Part model, mm, in its own coordinate system. A direction names the side the tool comes from. Coordinates: 2 decimals unless noted, no trailing zeros. Write each loop counter-clockwise with the first axis right and the second up, starting at its lowest first coordinate (ties: lowest second). Pieces come first, ordered by that corner, then holes. Notation, with made-up numbers: (-39.5, 54.5) -> (-4.5, 54.5) arc R21 ccw to (-4.5, 73.5) -> close; hole circle Ø6 at (74, -34). An arc over 180 degrees is marked (long way). Write item = value, one per line. Start each with the question number.
Q1. Band-saw the part on C-C, the plane z = 45. List the corners of the cut face in (x, y).
Q2. Probe line 1 (X direction, y = 49, z = 80); line 2 (Z direction, x = -56.35, y = 3.1); line 3 (Z direction, x = 35, y = 29.5). List the from-to ranges inside material, lowest first.
Q3. Band-saw the part on D-D, the plane y = 46.5. List the corners of the cut face in (x, z).
Q4. Band-saw the part on B-B, the plane x = -48. List the corners of the cut face in (y, z), plus the area to 3 significant figures.
Q5. Band-saw the part on A-A, the plane x = 56.35. List the corners of the cut face in (y, z).
Q6. Pull direction Z, two halves, no side cores. Call faces 1 (the flat face through (66.35, 2, 85)), 2 (the flat face through (-44, 4.947, 45)), 3 (the cylindrical face through (24.71, 37.73, 80.62)), 4 (the flat face through (-5, 42, 90)): released by +Z, released by -Z, zero draft, split by the parting line, or undercut.
Q7. Pin check, flat tips, straight feed: P1, Ø4, axis at y = 2, z = 43.5, coming from the +X side; P2, Ø7.5, axis at x = -20, z = 10, coming from the -Y side; P3, Ø11, axis at x = -55.5, z = 6.5, coming from the +Y side. Stop position of each tip, or through.
Q8. Tool access for faces 5 (the flat face through (41.35, 2, 45)), 6 (the flat face through (56, 3, 10)), 7 (the flat face through (-53.8, 5, 5.1)): list every direction of +Z, -Z, +X, -X, +Y, -Y with a clear straight run to the whole face (end or side of a thin tool).
from build123d import *

# Parameters (mm, degrees)
BOSS_EXTRUDE1_DEPTH      = 10
SKETCH2_W                = 10
SKETCH2_H                = 5
BOSS_EXTRUDE2_DEPTH      = 66.35
SKETCH3_R                = 2.3
CUT_EXTRUDE1_DEPTH       = 132.7
SKETCH4_R                = 41.35
CUT_EXTRUDE3_DEPTH       = 50
LPATTERN4_START          = 80
LPATTERN4_DEPTH          = 10
LPATTERN4_2_DEPTH        = 10
LPATTERN4_3_DEPTH        = 10
MIRROR5_COPY_1_SKETCH_R  = 2.3
MIRROR5_COPY_1_DEPTH     = 132.7
SKETCH8_W                = 4.648420871
SKETCH8_H                = 4.94728133
BOSS_EXTRUDE3_DEPTH      = 40
SKETCH11_W               = 60
SKETCH11_H               = 17
BOSS_EXTRUDE4_DEPTH      = 90
SKETCH12_R               = 41.35
CUT_EXTRUDE4_DEPTH       = 250
SKETCH14_R               = 2.3
CUT_EXTRUDE6_DEPTH       = 150
MIRROR8_COPY_1_SKETCH_R  = 2.3
MIRROR8_COPY_1_DEPTH     = 150
SKETCH15_R               = 9
CUT_EXTRUDE7_DEPTH       = 67
SKETCH16_W               = 5
SKETCH16_H               = 90
BOSS_EXTRUDE5_DEPTH      = 5
SKETCH18_R               = 4.75
CUT_EXTRUDE8_DEPTH       = 5
MIRROR10_COPY_1_SKETCH_R = 4.75
MIRROR10_COPY_1_DEPTH    = 5


# Read off the part's stored shape, not the designer's step: LPattern4
with BuildPart() as part:
    # Sketch1 → Boss-Extrude1 (new body)
    with BuildSketch(Plane.XY):
        with BuildLine():
            Line((-46.35, 0), (-41.35, 0))
            ThreePointArc((-41.35, 0), (0, 41.35), (41.35, 0))
            Line((41.35, 0), (46.35, 0))
            ThreePointArc((46.35, 0), (0, 46.35), (-46.35, 0))
        make_face()
    extrude(amount=BOSS_EXTRUDE1_DEPTH)



with BuildPart() as body_2:
    # Sketch2 → Boss-Extrude2 (new, symmetric)
    with BuildSketch(Plane(origin=(0, 0, 0), x_dir=(0, 0, -1), z_dir=(1, 0, 0))):
        with Locations((-5, 2.5)):
            Rectangle(SKETCH2_W, SKETCH2_H)
    extrude(amount=BOSS_EXTRUDE2_DEPTH, both=True)

    # Sketch3 → Cut-Extrude1 (cut)
    with BuildSketch(Plane(origin=(0, 5, 0), x_dir=(1, 0, 0), z_dir=(0, 1, 0))):
        with Locations(Location((56.35, -5, 0), (0, 0, 270))):
            Circle(SKETCH3_R)
    cut_extrude1 = extrude(amount=-CUT_EXTRUDE1_DEPTH, mode=Mode.SUBTRACT)

    # Mirror1: Cut-Extrude1 across plane
    add(cut_extrude1.mirror(Plane(origin=(0, 0, 0), x_dir=(0, 0, 1), z_dir=(1, 0, 0))), mode=Mode.SUBTRACT)

    # Sketch4 → Cut-Extrude3 (cut, symmetric)
    with BuildSketch(Plane.XY):
        Circle(SKETCH4_R)
    extrude(amount=CUT_EXTRUDE3_DEPTH, both=True, mode=Mode.SUBTRACT)


with BuildPart() as cut_extrude3_piece_1:
    # of the separate pieces the step leaves, piece 1, a body of its own (cut_extrude3_pieces)
    add(body_2.part.solids().sort_by_distance((-41.35, 0, 10))[0])


with BuildPart() as cut_extrude3_piece_2:
    # of the separate pieces the step leaves, piece 2, a body of its own (cut_extrude3_pieces)
    add(body_2.part.solids().sort_by_distance((66.35, 0, 10))[0])


with BuildPart() as body_4:
    # LPattern4 outline → LPattern4 (new body)
    with BuildSketch(Plane.XY.offset(LPATTERN4_START)):
        with BuildLine():
            Line((66.35, 0), (66.35, 5))
            Line((66.35, 5), (41.046589383, 5))
            ThreePointArc((41.046589383, 5), (41.274077646, 2.504598671), (41.35, 0))
            Line((41.35, 0), (66.35, 0))
        make_face()
    extrude(amount=LPATTERN4_DEPTH)

    # Mirror5: Cut-Extrude1 across plane
    add(cut_extrude1.mirror(Plane.XY.offset(45)), mode=Mode.SUBTRACT)


with BuildPart() as body_5:
    # LPattern4 2 outline → LPattern4 2 (new body)
    with BuildSketch(Plane.XY.offset(LPATTERN4_START)):
        with BuildLine():
            Line((-46.35, 0), (-41.35, 0))
            ThreePointArc((-41.35, 0), (0, 41.35), (41.35, 0))
            Line((41.35, 0), (46.35, 0))
            ThreePointArc((46.35, 0), (0, 46.35), (-46.35, 0))
        make_face()
    extrude(amount=LPATTERN4_2_DEPTH)


with BuildPart() as body_6:
    # LPattern4 3 outline → LPattern4 3 (new body)
    with BuildSketch(Plane.XY.offset(LPATTERN4_START)):
        with BuildLine():
            Line((-66.35, 0), (-41.35, 0))
            ThreePointArc((-41.35, 0), (-41.274077646, 2.504598671), (-41.046589383, 5))
            Line((-41.046589383, 5), (-66.35, 5))
            Line((-66.35, 5), (-66.35, 0))
        make_face()
    extrude(amount=LPATTERN4_3_DEPTH)

    # Mirror5 copy 1 sketch → Mirror5 copy 1 (cut)
    with BuildSketch(Plane(origin=(0, 5, 90), x_dir=(-1, 0, 0), z_dir=(0, 1, 0))):
        with Locations(Location((56.35, -5, 0), (0, 0, 270))):
            Circle(MIRROR5_COPY_1_SKETCH_R)
    extrude(amount=-MIRROR5_COPY_1_DEPTH, mode=Mode.SUBTRACT)


with BuildPart() as part_1:
    add(part.part)

    add(cut_extrude3_piece_1.part)  # Boss-Extrude3 merges Cut-Extrude3 piece 1

    add(body_5.part)  # Boss-Extrude3 merges body 5

    add(body_6.part)  # Boss-Extrude3 merges body 6
    # Sketch8 → Boss-Extrude3 (add, symmetric)
    with BuildSketch(Plane.XY.offset(45)):
        with Locations((-43.674210436, 2.473640665)):
            Rectangle(SKETCH8_W, SKETCH8_H)
    boss_extrude3 = extrude(amount=BOSS_EXTRUDE3_DEPTH, both=True)

    # Mirror6: Boss-Extrude3 across plane
    add(boss_extrude3.mirror(Plane(origin=(0, 0, 0), x_dir=(0, 0, 1), z_dir=(1, 0, 0))))

    # Sketch11 → Boss-Extrude4 (add)
    with BuildSketch(Plane.XY.offset(90)):
        with Locations((0, 44.255632839)):
            Rectangle(SKETCH11_W, SKETCH11_H)
    extrude(amount=-BOSS_EXTRUDE4_DEPTH)

    # Sketch12 → Cut-Extrude4 (cut, symmetric)
    with BuildSketch(Plane.XY.offset(90)):
        Circle(SKETCH12_R)
    extrude(amount=CUT_EXTRUDE4_DEPTH, both=True, mode=Mode.SUBTRACT)

    # Sketch14 → Cut-Extrude6 (cut, symmetric)
    with BuildSketch(Plane(origin=(0, 52.755632839, 0), x_dir=(1, 0, 0), z_dir=(0, 1, 0))):
        with Locations(Location((20, -80, 0), (0, 0, 270))):
            Circle(SKETCH14_R)
    cut_extrude6 = extrude(amount=CUT_EXTRUDE6_DEPTH, both=True, mode=Mode.SUBTRACT)

    # Mirror7: Cut-Extrude6 across plane
    add(cut_extrude6.mirror(Plane(origin=(0, 0, 0), x_dir=(0, 0, 1), z_dir=(1, 0, 0))), mode=Mode.SUBTRACT)

    # Mirror8: Cut-Extrude6 across plane
    add(cut_extrude6.mirror(Plane.XY.offset(45)), mode=Mode.SUBTRACT)

    # Mirror8 copy 1 sketch → Mirror8 copy 1 (cut, symmetric)
    with BuildSketch(Plane(origin=(0, 52.755632839, 90), x_dir=(-1, 0, 0), z_dir=(0, 1, 0))):
        with Locations(Location((20, -80, 0), (0, 0, 270))):
            Circle(MIRROR8_COPY_1_SKETCH_R)
    extrude(amount=MIRROR8_COPY_1_DEPTH, both=True, mode=Mode.SUBTRACT)

    # Sketch15 → Cut-Extrude7 (cut)
    with BuildSketch(Plane.ZY.offset(30)):
        with Locations((45, 52.755632839)):
            Circle(SKETCH15_R)
    extrude(amount=-CUT_EXTRUDE7_DEPTH, mode=Mode.SUBTRACT)


    add(cut_extrude3_piece_2.part)  # Boss-Extrude5 merges Cut-Extrude3 piece 2

    add(body_4.part)  # Boss-Extrude5 merges body 4
    # Sketch16 → Boss-Extrude5 (add)
    with BuildSketch(Plane.XZ):
        with Locations((43.85, 45)):
            Rectangle(SKETCH16_W, SKETCH16_H)
    extrude(amount=-BOSS_EXTRUDE5_DEPTH)

    # Sketch18 → Cut-Extrude8 (cut, symmetric)
    with BuildSketch(Plane.XZ.offset(-35.755632839)):
        with Locations(Location((20, 80, 0), (0, 0, 270))):
            Circle(SKETCH18_R)
    cut_extrude8 = extrude(amount=CUT_EXTRUDE8_DEPTH, both=True, mode=Mode.SUBTRACT)

    # Mirror9: Cut-Extrude8 across plane
    add(cut_extrude8.mirror(Plane.XY.offset(45)), mode=Mode.SUBTRACT)

    # Mirror10: Cut-Extrude8 across plane
    add(cut_extrude8.mirror(Plane(origin=(0, 0, 0), x_dir=(0, 0, 1), z_dir=(1, 0, 0))), mode=Mode.SUBTRACT)

    # Mirror10 copy 1 sketch → Mirror10 copy 1 (cut, symmetric)
    with BuildSketch(Plane(origin=(0, 35.755632839, 90), x_dir=(-1, 0, 0), z_dir=(0, -1, 0))):
        with Locations(Location((20, 80, 0), (0, 0, 270))):
            Circle(MIRROR10_COPY_1_SKETCH_R)
    extrude(amount=MIRROR10_COPY_1_DEPTH, both=True, mode=Mode.SUBTRACT)


solid = part_1.part
Ans:
q1.outline = (-46, 0) -> (-41.35, 0) -> (-41.35, 4.95) -> (-46, 4.95) -> close; (-30, 35.76) -> (-20.77, 35.76) arc R41.35 cw to (20.77, 35.76) -> (30, 35.76) -> (30, 43.76) -> (-30, 43.76) -> close; (41.35, 0) -> (46.35, 0) -> (46.35, 5) -> (41.35, 5) -> close
q2.line_1 = -30 to -22.3, -17.7 to 17.7, 22.3 to 30
q2.line_2 = 0 to 2.7, 7.3 to 10, 80 to 82.7, 87.3 to 90
q2.line_3 = 0 to 10, 80 to 90
q3.outline = (-30, 0) -> (30, 0) -> (30, 38.53) -> (-30, 38.53) -> close; (-30, 51.47) -> (30, 51.47) -> (30, 90) -> (-30, 90) -> close; hole circle Ø4.6 at (-20, 10); hole circle Ø4.6 at (-20, 80); hole circle Ø4.6 at (20, 10); hole circle Ø4.6 at (20, 80)
q4.outline = (0, 0) -> (5, 0) -> (5, 10) -> (0, 10) -> close; (0, 80) -> (5, 80) -> (5, 90) -> (0, 90) -> close
q4.area = 100 mm2
q5.outline = (0, 0) -> (5, 0) -> (5, 2.7) -> (0, 2.7) -> close; (0, 7.3) -> (5, 7.3) -> (5, 10) -> (0, 10) -> close; (0, 80) -> (5, 80) -> (5, 82.7) -> (0, 82.7) -> close; (0, 87.3) -> (5, 87.3) -> (5, 90) -> (0, 90) -> close
q6.face_1 = zero draft
q6.face_2 = undercut
q6.face_3 = undercut
q6.face_4 = released by +Z
q7.P1 = 46.35
q7.P2 = 40.76
q7.P3 = 5
q8.face_5 = +Y, -Y
q8.face_6 = +X, +Y, -Y
q8.face_7 = +Z, -Z, -X, +Y
